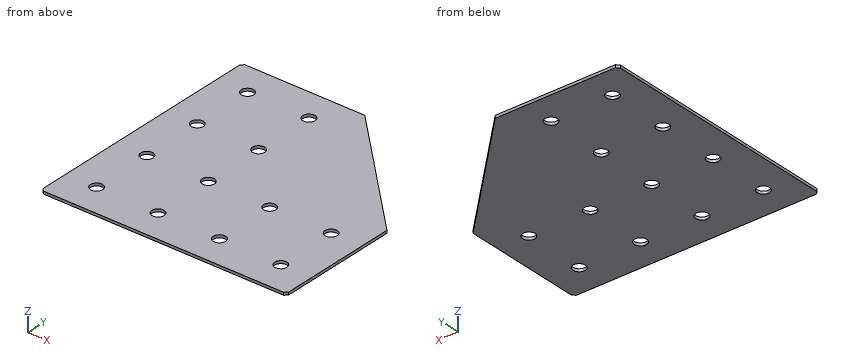
```python
from build123d import *

# Parameters (mm, degrees)
EXTRUDE_1_DEPTH   = 2
HOLE_WIZARD_M81_D = 9
CHAMFER_1_SIZE    = 2


with BuildPart() as part:
    # Эскиз1 → Бобышка-Вытянуть1 (new body)
    with BuildSketch(Plane(origin=(0, 0, 0), x_dir=(1, 0, 0), z_dir=(0, 0, -1))):
        Polygon((0, 0), (0, 180), (180, 180), (180, 90), (90, 0), align=None)
    extrude(amount=EXTRUDE_1_DEPTH)

    # Отверстие с зазором M81 (through all)
    with Locations(Plane(origin=(0, 0, -2), x_dir=(1, 0, 0), z_dir=(0, 0, -1))):
        with Locations((22.5, 157.5), (22.5, 112.5), (22.5, 67.5), (22.5, 22.5), (67.5, 157.5), (67.5, 112.5), (67.5, 67.5), (67.5, 22.5), (112.5, 157.5), (112.5, 112.5), (157.5, 157.5), (157.5, 112.5)):
            Hole(HOLE_WIZARD_M81_D / 2)

    # Фаска1
    chamfer_1_edges = [part.edges().sort_by_distance(p)[0] for p in [
        (0, 0, -1),
        (0, -180, -1),
        (180, -180, -1),
    ]]
    chamfer(chamfer_1_edges, length=CHAMFER_1_SIZE)


solid = part.part
```
Input: part model. Units: mm. Frame: model coordinates. Coordinates: 2 decimals unless noted, no trailing zeros. Write each loop counter-clockwise with the first axis right and the second up, starting at its lowest first coordinate (ties: lowest second). Pieces come first, ordered by that corner, then holes.
1) Section A-A on y = -67.5. Output: boundary loops of the cut face in (x, z), and give its area (3 significant figures).
2) Section B-B on x = 112.5. Output: boundary loops of the cut face in (y, z), and give its area (3 significant figures).
3) Material intervals for line 1 along X through (y, z) = (-157.5, -1.3); line 2 along Y through (x, z) = (67.5, -1.05); line 3 along Y through (x, z) = (157.5, -0.7), sorted ascending.
4) Section D-D on y = -112.5. Output: boundary loops of the cut face in (x, z).
5) Section C-C on z = -0.6. State how many separate pieces and enclosed holes the cut face has, and give its area (3 significant figures).
6) Pin query (flat end, axial travel): pin 1 Ø5.5 at (x, y) = (67.5, -157.5) entering from +Z. Return the tip coordinate at first contact, or that it passes through.
Check result:
1. outline: (0, -2) - (18, -2) - (18, 0) - (0, 0) - close; (27, -2) - (63, -2) - (63, 0) - (27, 0) - close; (72, -2) - (157.5, -2) - (157.5, 0) - (72, 0) - close
1. area: 279 mm2
2. outline: (-180, -2) - (-162, -2) - (-162, 0) - (-180, 0) - close; (-153, -2) - (-117, -2) - (-117, 0) - (-153, 0) - close; (-108, -2) - (-22.5, -2) - (-22.5, 0) - (-108, 0) - close
2. area: 279 mm2
3. line 1: x = 0 to 18, 27 to 63, 72 to 108, 117 to 153, 162 to 180
3. line 2: y = -180 to -162, -153 to -117, -108 to -72, -63 to -27, -18 to 0
3. line 3: y = -180 to -162, -153 to -117, -108 to -67.5
4. outline: (0, -2) - (18, -2) - (18, 0) - (0, 0) - close; (27, -2) - (63, -2) - (63, 0) - (27, 0) - close; (72, -2) - (108, -2) - (108, 0) - (72, 0) - close; (117, -2) - (153, -2) - (153, 0) - (117, 0) - close; (162, -2) - (180, -2) - (180, 0) - (162, 0) - close
5. separate pieces: 1
5. enclosed holes: 12
5. area: 27,600 mm2
6. pin 1: passes through
